Input: part model. Units: mm. Frame: model coordinates. A direction names the side the tool comes from. Coordinates: 2 decimals unless noted, no trailing zeros. Write each loop counter-clockwise with the first axis right and the second up, starting at its lowest first coordinate (ties: lowest second). Pieces come first, ordered by that corner, then holes. Notation, with made-up numbers: M -25,-37 L -13,-37 A18 ccw -13,-31 Z; hole C -4,69.5 d3. An arc over 180 degrees is marked long. Use CSV: the item, a comma, the result in double quotes.
```python
from build123d import *

# Parameters (mm, degrees)
SKETCH1_R               = 10.95
SKETCH1_R_2             = 10.05
BOSS_EXTRUDE1_DEPTH     = 2
BOSS_EXTRUDE2_START     = 15
SKETCH1_3_R             = 10.95
SKETCH1_3_R_2           = 10.05
BOSS_EXTRUDE2_DEPTH     = 15
BOSS_EXTRUDE3_START     = -2.5
SKETCH2_R               = 12.95
SKETCH2_R_2             = 10.95
BOSS_EXTRUDE3_DEPTH     = 14.5
CUT_EXTRUDE1_DEPTH      = 24.672874773
CUT_EXTRUDE1_DEPTH_BACK = 24.672874773
SKETCH3_W               = 100
SKETCH3_H               = 24
CUT_EXTRUDE3_DEPTH      = 24.166840527
CUT_EXTRUDE3_DEPTH_BACK = 24.166840527
BOSS_EXTRUDE4_START     = 15
SKETCH1_4_R             = 10.95
SKETCH1_4_R_2           = 10.05
BOSS_EXTRUDE4_DEPTH     = 15
SKETCH5_W               = 18
SKETCH5_H               = 4
CUT_EXTRUDE4_DEPTH      = 24.166840527
FILLET1_R               = 2
FILLET2_R               = 4
CUT_EXTRUDE5_DEPTH      = 24.166840699
CUT_EXTRUDE5_DEPTH_BACK = 24.166840699
SKETCH6_R               = 1.6


with BuildPart() as part:
    # Sketch1 → Boss-Extrude1 (new body)
    # profile 1 of 2: a face of its own
    with BuildSketch(Plane(origin=(0, 0, 0), x_dir=(1, 0, 0), z_dir=(0, 1, 0))):
        with Locations(Location((0, 0, 0), (0, 0, 270))):
            Circle(SKETCH1_R)
        Circle(SKETCH1_R_2, mode=Mode.SUBTRACT)
    # profile 2 of 2: a face of its own
    with BuildSketch(Plane(origin=(0, 0, 0), x_dir=(1, 0, 0), z_dir=(0, 1, 0))):
        Circle(SKETCH1_R_2)
    extrude(amount=-BOSS_EXTRUDE1_DEPTH)

    # Sketch1<3> → Boss-Extrude2 (add)
    with BuildSketch(Plane(origin=(0, 0, 0), x_dir=(1, 0, 0), z_dir=(0, 1, 0)).offset(BOSS_EXTRUDE2_START)):
        with Locations(Location((0, 0, 0), (0, 0, 270))):
            Circle(SKETCH1_3_R)
        with Locations(Location((0, 0, 0), (0, 0, 270))):
            Circle(SKETCH1_3_R_2, mode=Mode.SUBTRACT)
    extrude(amount=-BOSS_EXTRUDE2_DEPTH)

    # Sketch2 → Boss-Extrude3 (add)
    with BuildSketch(Plane(origin=(0, 15, 0), x_dir=(1, 0, 0), z_dir=(0, 1, 0)).offset(BOSS_EXTRUDE3_START)):
        with Locations(Location((0, 0, 0), (0, 0, 270))):
            Circle(SKETCH2_R)
        with Locations(Location((0, 0, 0), (0, 0, 270))):
            Circle(SKETCH2_R_2, mode=Mode.SUBTRACT)
    extrude(amount=-BOSS_EXTRUDE3_DEPTH)

    # Sketch3 → Cut-Extrude1 (cut, two sides: drawn at the far end of the back side and taken through both)
    with BuildSketch(Plane(origin=(0, 0, 0), x_dir=(1, 0, 0), z_dir=(0, 1, 0)).offset(-CUT_EXTRUDE1_DEPTH_BACK)):
        with Locations((0, -24)):
            Rectangle(SKETCH3_W, SKETCH3_H)
        with Locations((0, 24)):
            Rectangle(SKETCH3_W, SKETCH3_H)
    extrude(amount=CUT_EXTRUDE1_DEPTH + CUT_EXTRUDE1_DEPTH_BACK, mode=Mode.SUBTRACT)

    # Sketch4 → Cut-Extrude3 (cut, two sides: drawn at the far end of the back side and taken through both)
    with BuildSketch(Plane.XY.offset(-CUT_EXTRUDE3_DEPTH_BACK)):
        Polygon((13, 15), (5, 15), (13, 7), align=None)
    extrude(amount=CUT_EXTRUDE3_DEPTH + CUT_EXTRUDE3_DEPTH_BACK, mode=Mode.SUBTRACT)

    # Sketch1<4> → Boss-Extrude4 (add)
    with BuildSketch(Plane(origin=(0, 0, 0), x_dir=(1, 0, 0), z_dir=(0, 1, 0)).offset(BOSS_EXTRUDE4_START)):
        with Locations(Location((0, 0, 0), (0, 0, 270))):
            Circle(SKETCH1_4_R)
        with Locations(Location((0, 0, 0), (0, 0, 270))):
            Circle(SKETCH1_4_R_2, mode=Mode.SUBTRACT)
    extrude(amount=-BOSS_EXTRUDE4_DEPTH)

    # Sketch5 → Cut-Extrude4 (cut, through all)
    with BuildSketch(Plane(origin=(0, 0, 0), x_dir=(1, 0, 0), z_dir=(0, 1, 0))):
        with Locations((-11, 0)):
            Rectangle(SKETCH5_W, SKETCH5_H)
    extrude(amount=CUT_EXTRUDE4_DEPTH, mode=Mode.SUBTRACT)

    # Fillet1
    fillet1_edges = [part.edges().sort_by_distance(p)[0] for p in [
        (-10.307393529, 15, 2),
        (-10.307393529, 15, -2),
        (-11.321806249, 0, -2),
        (-11.321806249, 0, 2),
    ]]
    fillet(fillet1_edges, radius=FILLET1_R - 0.0001)  # a hair under: the kernel refuses the full size

    # Fillet2
    fillet2_edges = [part.edges().sort_by_distance(p)[0] for p in [
        (7.5, 12.5, 9.26767915),
        (7.5, 12.5, -9.26767915),
    ]]
    fillet(fillet2_edges, radius=FILLET2_R)

    # Sketch6 → Cut-Extrude5 (cut, two sides: drawn at the far end of the back side and taken through both)
    with BuildSketch(Plane(origin=(0, 0, 0), x_dir=(1, 0, 0), z_dir=(0, 1, 0)).offset(-CUT_EXTRUDE5_DEPTH_BACK)):
        with Locations(Location((0, 0, 0), (0, 0, 270))):
            Circle(SKETCH6_R)
    extrude(amount=CUT_EXTRUDE5_DEPTH + CUT_EXTRUDE5_DEPTH_BACK, mode=Mode.SUBTRACT)


solid = part.part
```
1. Section D-D (x = 6.5). Return loops of the section in (y, z).
Resolved:
outline,"M -2,-11.2 L 12.45,-11.2 L 12.45,-8.81 L 15,-8.81 L 15,-7.67 L 0,-7.67 L 0,7.67 L 15,7.67 L 15,8.81 L 12.45,8.81 L 12.45,11.2 L -2,11.2 Z"
2. Contact query for flat-ended pins moving along their axis: pin 1 Ø2.5 at (x, y) = (-11.5, 9) entering from +Z; pin 2 Ø6 at (x, y) = (9.5, 0.5) entering from -Z; pin 3 Ø8 at (x, z) = (0.5, 5) entering from +Y. Output: stop coordinate, or through.
Resolved:
pin 1,"stops at z = 7.91"
pin 2,"stops at z = -11.2"
pin 3,"stops at y = 0"
3. Section B-B (y = 4.25). Return loops of the section in (x, z).
Resolved:
outline,"M -12.79,-2 A12.95 ccw -4.87,-12 L 4.87,-12 A12.95 ccw 4.87,12 L -4.87,12 A12.95 ccw -12.79,2 L -9.85,2 A10.05 cw long -9.85,-2 Z"
4. Access query for faces 1 (the cylindrical face through (7.39, 12.19, -9.16)), 2 (the cylindrical face through (7.39, 12.19, 9.09)), 3 (the flat face through (-11, 7, 2)), 4 (the flat face through (0, -2, 2)), 5 (the flat face through (-2, 0, 0)). Directions: +Z, -Z, +X, -X, +Y, -Y. A direction counts if a zero-diameter tool reaches every point of the face in a straight line with its end or side. Return the directions, or none.
Resolved:
face 1,"-Z, +X, +Y"
face 2,"+Z, +X, +Y"
face 3,"-X, +Y"
face 4,"+Z, -Z, +X, -X, -Y"
face 5,"+Y"
5. Material intervals for line 1 (X direction, y = -0.7, z = 0); line 2 (Z direction, x = 0, y = -1.35); line 3 (Z direction, x = 0, y = 11.75), sorted ascending. Write a range as [from, to].
Resolved:
line 1,"x = [-12.95, -1.6], [1.6, 12.95]"
line 2,"z = [-12, -1.6], [1.6, 12]"
line 3,"z = [-12, -10.05], [10.05, 12]"
6. Section A-A (x = 0). Return loops of the section in (y, z), then the cut area to 4 significant figures.
Resolved:
outline,"M -2,-12 L 12.5,-12 L 12.5,-10.95 L 15,-10.95 L 15,-10.05 L 0,-10.05 L 0,-1.6 L -2,-1.6 Z; M -2,1.6 L 0,1.6 L 0,10.05 L 15,10.05 L 15,10.95 L 12.5,10.95 L 12.5,12 L -2,12 Z"
area,"94.85 mm^2"
7. Section C-C (z = -5.5). Return loops of the section in (x, y), then the cut area to 3 significant figures.
Resolved:
outline,"M -11.72,-2 L 11.72,-2 L 11.72,8.28 L 9.47,10.53 L 9.47,15 L 8.41,15 L 8.41,0 L -8.41,0 L -8.41,15 L -9.47,15 L -9.47,12.5 L -11.72,12.5 Z"
area,"128 mm^2"
8. Mould query, pull axis X, two halves, no side actions, for faces 6 (the flat face through (11.3, 8.7, -0.1)), 7 (the cylindrical face through (-0.97, -1.01, -1.27)), 8 (the cylindrical face through (10.94, 13.3, 0.45)), 9 (the cylindrical face through (-11.38, 0.57, 1.4)). Classes: pulls with the +X half, pulls with the -X half, needs draft (parallel to the pull), parting line crosses it, or undercut.
Resolved:
face 6,"pulls with the +X half"
face 7,"undercut"
face 8,"parting line crosses it"
face 9,"needs draft"
